Read the model definition and answer for the solid it produces. Units are mm, in the model's axes. A direction names the side the tool comes from. Give positions to 0.01 mm unless a question says otherwise; leave off trailing zeros. Loops run counter-clockwise (first coordinate to the right, second up) from the corner with the lowest first, then second, coordinate; pieces in that order, holes last.
(1) Find section B-B, the plane y = 10.5. Write down the section's boundary in (x, z).
(2) Determine the mould class of faces 3 (the face through (0, 17, 1)), 4 (the face through (-5.037, 9.93, -12.147)), 5 (the face through (13.1, 15, -2.4)) for opening direction X: pulls with the +X half, pulls with the -X half, needs draft (parallel to the pull), parting line crosses it, or undercut.
(3) Find section C-C, the plane x = -11.5. Write down the section's boundary in (y, z).
(4) Find section D-D, the plane z = 6. Write down the section's boundary in (x, y), then the cut area to 3 significant figures.
(5) Which of the six approach directions +Z, -Z, +X, -X, +Y, -Y give full straight-line access (tool end or side, diameter ignored) to faces 1 (the face through (3, 15, -2)), 2 (the face through (-15.62, 16.23, -3.47))?
(6) Each of these flat-tipped pins is pushed along its axis until it touches: P1, Ø6, axis at y = 13, z = 4.5, coming from the +X side; P2, Ø6, axis at y = 7.5, z = 7.5, coming from the -X side; P3, Ø1, axis at x = 4, z = 7.5, coming from the -Y side. Where does it stop, or does it pass through?
(7) Straight lines are drawn through the part: probe 1 along X at (y, z) = (13.8, 0); probe 2 along Y at (x, z) = (8, 11); probe 3 along Z at (x, y) = (6, 12). For each, find the intervals that lie inside material, in ascending order.
(8) Find section A-A, the plane z = 12.5. Write down the section's boundary in (x, y).
```python
from build123d import *

# Parameters (mm, degrees)
SKETCH1_R           = 12.65
SKETCH1_R_2         = 10.65
BOSS_EXTRUDE1_DEPTH = 15
SKETCH2_R           = 16
BOSS_EXTRUDE2_DEPTH = 2
CUT_EXTRUDE2_DEPTH  = 3.3
SKETCH5_R           = 16
BOSS_EXTRUDE4_DEPTH = 0.5
SKETCH7_R           = 13.15
SKETCH7_R_2         = 12.65
BOSS_EXTRUDE5_DEPTH = 15
BOSS_EXTRUDE6_DEPTH = 2
SKETCH10_R          = 13.15
CUT_EXTRUDE3_DEPTH  = 5
SKETCH11_R          = 10.65
CUT_EXTRUDE4_DEPTH  = 2


with BuildPart() as part:
    # Sketch1 → Boss-Extrude1 (new body)
    with BuildSketch(Plane(origin=(0, 0, 0), x_dir=(1, 0, 0), z_dir=(0, 1, 0))):
        with Locations(Location((0, 0, 0), (0, 0, 270))):
            Circle(SKETCH1_R)
        with Locations(Location((0, 0, 0), (0, 0, 270))):
            Circle(SKETCH1_R_2, mode=Mode.SUBTRACT)
    extrude(amount=BOSS_EXTRUDE1_DEPTH)

    # Sketch2 → Boss-Extrude2 (add)
    with BuildSketch(Plane(origin=(0, 15, 0), x_dir=(1, 0, 0), z_dir=(0, 1, 0))):
        with Locations(Location((0, 0, 0), (0, 0, 270))):
            Circle(SKETCH2_R)
    extrude(amount=BOSS_EXTRUDE2_DEPTH)

    # Sketch4 → Cut-Extrude2 (cut)
    with BuildSketch(Plane(origin=(0, 17, 0), x_dir=(1, 0, 0), z_dir=(0, 1, 0))):
        with BuildLine():
            ThreePointArc((-7.706902754, 1.808391197), (-7.603132783, 1.898306548), (-7.527733553, 2.013058165))
            add(Edge.make_bspline(
                [(-5.973562898, 3.427644412), (-6.705514393, 3.181828062), (-7.188037686, 2.727956598), (-7.527733553, 2.013058165)],
                knots=[0.175947617, 0.175947617, 0.175947617, 0.175947617, 0.967261409, 0.967261409, 0.967261409, 0.967261409], degree=3))
            ThreePointArc((-5.973562898, 3.427644412), (-5.5249107, 3.522844059), (-5.066368092, 3.513333887))
            add(Edge.make_bspline(
                [(0.252246957, 2.546498923), (-0.967265157, 2.585544634), (-2.911735898, 3.219251878), (-5.066368092, 3.513333887)],
                knots=[0, 0, 0, 0, 0.944652434, 0.944652434, 0.944652434, 0.944652434], degree=3))
            add(Edge.make_bspline(
                [(2.984843767, 2.898010668), (1.699544821, 2.557369315), (0.252246957, 2.546498923)],
                knots=[0, 0, 0, 1, 1, 1], degree=2))
            add(Edge.make_bspline(
                [(1.446576088, 1.819612756), (1.692233604, 2.009446504), (2.255675441, 2.356061237), (2.984843767, 2.898010668)],
                knots=[0.144955644, 0.144955644, 0.144955644, 0.144955644, 1, 1, 1, 1], degree=3))
            ThreePointArc((1.446576088, 1.819612756), (1.407722351, 1.740462389), (1.446612546, 1.661329929))
            add(Edge.make_bspline(
                [(10.133171434, -3.748192499), (7.984235622, -2.549090336), (4.381903984, -0.604779848), (1.446612546, 1.661329929)],
                knots=[0.010904337, 0.010904337, 0.010904337, 0.010904337, 1, 1, 1, 1], degree=3))
            Line((10.133171434, -3.748192499), (-3.273421479, -3.865089106))
            add(Edge.make_bspline(
                [(-7.527733553, 0.078549357), (-6.021351328, 0.034537537), (-5.034172952, -1.161131544), (-3.273421479, -3.865089106)],
                knots=[0, 0, 0, 0, 1, 1, 1, 1], degree=3))
            add(Edge.make_bspline(
                [(-9.001359598, -0.096644929), (-8.609511327, -0.010984191), (-8.147442934, 0.043060836), (-7.527733553, 0.078549357)],
                knots=[0.366671919, 0.366671919, 0.366671919, 0.366671919, 1, 1, 1, 1], degree=3))
            ThreePointArc((-9.001359598, -0.096644929), (-9.440291534, -0.378150341), (-9.589622684, -0.877756935))
            Line((-9.589622684, -0.877756935), (-9.555879634, -1.399381307))
            Line((-9.555879634, -1.399381307), (-10.239201334, 0.078549357))
            ThreePointArc((-10.239201334, 0.078549357), (-10.259690649, 0.446534823), (-10.022461777, 0.728590805))
            add(Edge.make_bspline(
                [(-7.706902754, 1.808391197), (-8.132820465, 1.531622413), (-9.295077766, 1.120365549), (-10.022461777, 0.728590805)],
                knots=[0.10934646, 0.10934646, 0.10934646, 0.10934646, 0.840811763, 0.840811763, 0.840811763, 0.840811763], degree=3))
        make_face()
        with BuildLine():
            add(Edge.make_bspline(
                [(-6.583224352, 1.672229032), (-6.265045802, 1.812995825), (-5.554174981, 1.756337096)],
                knots=[0, 0, 0, 1, 1, 1], degree=2))
            ThreePointArc((-5.554174981, 1.756337096), (-5.456989048, 1.782455761), (-5.398182511, 1.864120205))
            add(Edge.make_bspline(
                [(-5.398182511, 1.864120205), (-5.299215588, 2.205704199), (-5.024689184, 2.452345347)],
                knots=[0, 0, 0, 1, 1, 1], degree=2))
            add(Edge.make_bspline(
                [(-5.024689184, 2.452345347), (-5.951430889, 2.228368239), (-6.944366579, 2.126753853)],
                knots=[0, 0, 0, 1, 1, 1], degree=2))
            add(Edge.make_bspline(
                [(-6.944366579, 2.126753853), (-6.855792408, 2.003769494), (-6.788085292, 1.768000929)],
                knots=[0, 0, 0, 1, 1, 1], degree=2))
            ThreePointArc((-6.788085292, 1.768000929), (-6.707437973, 1.673519717), (-6.583224352, 1.672229032))
        make_face(mode=Mode.SUBTRACT)
        with BuildLine():
            ThreePointArc((-6.788085292, 1.768000929), (-6.707437973, 1.673519717), (-6.583224352, 1.672229032))
            add(Edge.make_bspline(
                [(-6.583224352, 1.672229032), (-6.265045802, 1.812995825), (-5.554174981, 1.756337096)],
                knots=[0, 0, 0, 1, 1, 1], degree=2))
            ThreePointArc((-5.554174981, 1.756337096), (-5.456989048, 1.782455761), (-5.398182511, 1.864120205))
            add(Edge.make_bspline(
                [(-5.398182511, 1.864120205), (-5.299215588, 2.205704199), (-5.024689184, 2.452345347)],
                knots=[0, 0, 0, 1, 1, 1], degree=2))
            add(Edge.make_bspline(
                [(-5.024689184, 2.452345347), (-5.951430889, 2.228368239), (-6.944366579, 2.126753853)],
                knots=[0, 0, 0, 1, 1, 1], degree=2))
            add(Edge.make_bspline(
                [(-6.944366579, 2.126753853), (-6.855792408, 2.003769494), (-6.788085292, 1.768000929)],
                knots=[0, 0, 0, 1, 1, 1], degree=2))
        make_face()
    extrude(amount=-CUT_EXTRUDE2_DEPTH, mode=Mode.SUBTRACT)

    # Sketch5 → Boss-Extrude4 (add)
    with BuildSketch(Plane(origin=(0, 17, 0), x_dir=(1, 0, 0), z_dir=(0, 1, 0))):
        with Locations(Location((0, 0, 0), (0, 0, 270))):
            Circle(SKETCH5_R)
    extrude(amount=BOSS_EXTRUDE4_DEPTH)

    # Sketch7 → Boss-Extrude5 (add)
    with BuildSketch(Plane.XZ):
        with Locations(Location((0, 0, 0), (0, 0, 270))):
            Circle(SKETCH7_R)
        Circle(SKETCH7_R_2, mode=Mode.SUBTRACT)
    extrude(amount=-BOSS_EXTRUDE5_DEPTH)

    # Sketch8 → Boss-Extrude6 (add)
    with BuildSketch(Plane.XZ.offset(-15)):
        with BuildLine():
            add(Edge.make_bspline(
                [(9.996866834, 3.672213707), (10.042920822, 3.697861429), (10.088362097, 3.723188972), (10.133171434, 3.748192499)],
                knots=[0.979375502, 0.979375502, 0.979375502, 0.979375502, 1, 1, 1, 1], degree=3))
            Line((10.133171434, 3.748192499), (9.9680871, 3.749631925))
            Line((9.9680871, 3.749631925), (-3.273421479, 3.865089106))
            add(Edge.make_bspline(
                [(-3.273421479, 3.865089106), (-5.034172952, 1.161131544), (-6.021351328, -0.034537537), (-7.527733553, -0.078549357)],
                knots=[0, 0, 0, 0, 1, 1, 1, 1], degree=3))
            add(Edge.make_bspline(
                [(-7.527733553, -0.078549357), (-8.147442934, -0.043060836), (-8.609511327, 0.010984191), (-9.001359598, 0.096644929)],
                knots=[0.366671919, 0.366671919, 0.366671919, 0.366671919, 1, 1, 1, 1], degree=3))
            ThreePointArc((-9.001359598, 0.096644929), (-9.440291534, 0.378150341), (-9.589622684, 0.877756935))
            Line((-9.589622684, 0.877756935), (-9.555879634, 1.399381307))
            Line((-9.555879634, 1.399381307), (-10.239201334, -0.078549357))
            ThreePointArc((-10.239201334, -0.078549357), (-10.259690649, -0.446534823), (-10.022461777, -0.728590805))
            add(Edge.make_bspline(
                [(-10.022461777, -0.728590805), (-9.295077766, -1.120365549), (-8.132820465, -1.531622413), (-7.706902754, -1.808391197)],
                knots=[0.10934646, 0.10934646, 0.10934646, 0.10934646, 0.840811763, 0.840811763, 0.840811763, 0.840811763], degree=3))
            ThreePointArc((-7.706902754, -1.808391197), (-7.603132783, -1.898306548), (-7.527733553, -2.013058165))
            add(Edge.make_bspline(
                [(-7.527733553, -2.013058165), (-7.188037686, -2.727956598), (-6.705514393, -3.181828062), (-5.973562898, -3.427644412)],
                knots=[0.175947617, 0.175947617, 0.175947617, 0.175947617, 0.967261409, 0.967261409, 0.967261409, 0.967261409], degree=3))
            ThreePointArc((-5.973562898, -3.427644412), (-5.5249107, -3.522844059), (-5.066368092, -3.513333887))
            add(Edge.make_bspline(
                [(-5.066368092, -3.513333887), (-2.911735898, -3.219251878), (-0.967265157, -2.585544634), (0.252246944, -2.546498923)],
                knots=[0, 0, 0, 0, 0.944652434, 0.944652434, 0.944652434, 0.944652434], degree=3))
            add(Edge.make_bspline(
                [(0.252246944, -2.546498923), (1.699544832, -2.557369314), (2.984843797, -2.898010676)],
                knots=[0, 0, 0, 1, 1, 1], degree=2))
            add(Edge.make_bspline(
                [(2.984843797, -2.898010676), (2.255675441, -2.356061237), (1.692233604, -2.009446504), (1.446576086, -1.819612759)],
                knots=[0.144955644, 0.144955644, 0.144955644, 0.144955644, 1, 1, 1, 1], degree=3))
            ThreePointArc((1.446576086, -1.819612759), (1.407722347, -1.740462389), (1.446612544, -1.661329926))
            add(Edge.make_bspline(
                [(1.446612544, -1.661329926), (4.320697658, 0.557527214), (7.834294925, 2.467865384), (9.996866834, 3.672213707)],
                knots=[0.010904337, 0.010904337, 0.010904337, 0.010904337, 0.979375502, 0.979375502, 0.979375502, 0.979375502], degree=3))
        make_face()
        with BuildLine():
            Line((-3.273421479, 3.865089106), (9.9680871, 3.749631925))
            ThreePointArc((9.9680871, 3.749631925), (-9.982552018, -3.710950716), (9.996866834, 3.672213707))
            add(Edge.make_bspline(
                [(1.446612544, -1.661329926), (4.320697658, 0.557527214), (7.834294925, 2.467865384), (9.996866834, 3.672213707)],
                knots=[0.010904337, 0.010904337, 0.010904337, 0.010904337, 0.979375502, 0.979375502, 0.979375502, 0.979375502], degree=3))
            ThreePointArc((1.446612544, -1.661329926), (1.407722347, -1.740462389), (1.446576086, -1.819612759))
            add(Edge.make_bspline(
                [(2.984843797, -2.898010676), (2.255675441, -2.356061237), (1.692233604, -2.009446504), (1.446576086, -1.819612759)],
                knots=[0.144955644, 0.144955644, 0.144955644, 0.144955644, 1, 1, 1, 1], degree=3))
            add(Edge.make_bspline(
                [(0.252246944, -2.546498923), (1.699544832, -2.557369314), (2.984843797, -2.898010676)],
                knots=[0, 0, 0, 1, 1, 1], degree=2))
            add(Edge.make_bspline(
                [(-5.066368092, -3.513333887), (-2.911735898, -3.219251878), (-0.967265157, -2.585544634), (0.252246944, -2.546498923)],
                knots=[0, 0, 0, 0, 0.944652434, 0.944652434, 0.944652434, 0.944652434], degree=3))
            ThreePointArc((-5.066368092, -3.513333887), (-5.5249107, -3.522844059), (-5.973562898, -3.427644412))
            add(Edge.make_bspline(
                [(-7.527733553, -2.013058165), (-7.188037686, -2.727956598), (-6.705514393, -3.181828062), (-5.973562898, -3.427644412)],
                knots=[0.175947617, 0.175947617, 0.175947617, 0.175947617, 0.967261409, 0.967261409, 0.967261409, 0.967261409], degree=3))
            ThreePointArc((-7.527733553, -2.013058165), (-7.603132783, -1.898306548), (-7.706902754, -1.808391197))
            add(Edge.make_bspline(
                [(-10.022461777, -0.728590805), (-9.295077766, -1.120365549), (-8.132820465, -1.531622413), (-7.706902754, -1.808391197)],
                knots=[0.10934646, 0.10934646, 0.10934646, 0.10934646, 0.840811763, 0.840811763, 0.840811763, 0.840811763], degree=3))
            ThreePointArc((-10.022461777, -0.728590805), (-10.259690649, -0.446534823), (-10.239201334, -0.078549357))
            Line((-10.239201334, -0.078549357), (-9.555879634, 1.399381307))
            Line((-9.555879634, 1.399381307), (-9.589622684, 0.877756935))
            ThreePointArc((-9.589622684, 0.877756935), (-9.440291534, 0.378150341), (-9.001359598, 0.096644929))
            add(Edge.make_bspline(
                [(-7.527733553, -0.078549357), (-8.147442934, -0.043060836), (-8.609511327, 0.010984191), (-9.001359598, 0.096644929)],
                knots=[0.366671919, 0.366671919, 0.366671919, 0.366671919, 1, 1, 1, 1], degree=3))
            add(Edge.make_bspline(
                [(-3.273421479, 3.865089106), (-5.034172952, 1.161131544), (-6.021351328, -0.034537537), (-7.527733553, -0.078549357)],
                knots=[0, 0, 0, 0, 1, 1, 1, 1], degree=3))
        make_face()
    extrude(amount=BOSS_EXTRUDE6_DEPTH)

    # Sketch10 → Cut-Extrude3 (cut)
    with BuildSketch(Plane.XZ):
        with Locations(Location((0, 0, 0), (0, 0, 270))):
            Circle(SKETCH10_R)
    extrude(amount=-CUT_EXTRUDE3_DEPTH, mode=Mode.SUBTRACT)

    # Sketch11 → Cut-Extrude4 (cut)
    with BuildSketch(Plane.XZ.offset(-13)):
        with Locations(Location((0, 0, 0), (0, 0, 270))):
            Circle(SKETCH11_R)
    extrude(amount=-CUT_EXTRUDE4_DEPTH, mode=Mode.SUBTRACT)


solid = part.part
```
Entries:
1. outline: circle Ø26.3 at (0, 0); hole circle Ø21.3 at (0, 0)
2. face 3: undercut
2. face 4: parting line crosses it
2. face 5: needs draft
3. outline: (5, -6.38) - (15, -6.38) - (15, -11.12) - (17.5, -11.12) - (17.5, 11.12) - (15, 11.12) - (15, 6.38) - (5, 6.38) - close
4. outline: (-14.83, 15) - (-11.7, 15) - (-11.7, 5) - (-8.8, 5) - (-8.8, 15) - (8.8, 15) - (8.8, 5) - (11.7, 5) - (11.7, 15) - (14.83, 15) - (14.83, 17.5) - (-14.83, 17.5) - close
4. area: 132 mm2
5. face 1: -Y
5. face 2: +Y, -Y
6. P1: stops at x = 15.84
6. P2: stops at x = -12.36
6. P3: stops at y = 15
7. probe 1: x = -13.15 to -10.65, 10.65 to 13.15
7. probe 2: y = 15 to 17.5
7. probe 3: z = -11.7 to -8.8, 8.8 to 11.7
8. outline: (-9.99, 15) - (-4.08, 15) - (-4.08, 5) - (4.08, 5) - (4.08, 15) - (9.99, 15) - (9.99, 17.5) - (-9.99, 17.5) - close
